```python
from build123d import *

# Parameters (mm, degrees)
SKETCH1_R           = 88.9
BOSS_EXTRUDE1_DEPTH = 76.2
CUT_EXTRUDE1_REACH  = 149.013


with BuildPart() as part:
    # Sketch1 → Boss-Extrude1 (new body)
    with BuildSketch(Plane.XY):
        with Locations(Location((0, 0, 0), (0, 0, 180))):
            Circle(SKETCH1_R)
    extrude(amount=BOSS_EXTRUDE1_DEPTH)

    # Sketch3 → Cut-Extrude1 (cut, up to next)
    with BuildSketch(Plane.XY.offset(76.2), mode=Mode.PRIVATE) as cut_extrude1_sk1:
        with BuildLine():
            Line((35.802288852, 13.030967461), (69.049928483, 32.226501152))
            ThreePointArc((69.049928483, 32.226501152), (74.391009371, 16.505081787), (76.2, 0))
            Line((76.2, 0), (38.1, 0))
            ThreePointArc((38.1, 0), (37.52117539, 6.615995569), (35.802288852, 13.030967461))
        make_face()
    cut_extrude1_tool1 = extrude(cut_extrude1_sk1.sketch, amount=-CUT_EXTRUDE1_REACH, mode=Mode.PRIVATE) & part.part
    # Sketch3 → Cut-Extrude1 (cut, up to next)
    with BuildSketch(Plane.XY.offset(76.2), mode=Mode.PRIVATE) as cut_extrude1_sk2:
        with BuildLine():
            Line((32.51038259, -19.866681249), (68.247619398, -33.892513133))
            ThreePointArc((68.247619398, -33.892513133), (59.286228254, -47.870482966), (47.509922902, -59.575558964))
            Line((47.509922902, -59.575558964), (23.754961451, -29.787779482))
            ThreePointArc((23.754961451, -29.787779482), (28.566663833, -25.210230412), (32.51038259, -19.866681249))
        make_face()
    cut_extrude1_tool2 = extrude(cut_extrude1_sk2.sketch, amount=-CUT_EXTRUDE1_REACH, mode=Mode.PRIVATE) & part.part
    # Sketch3 → Cut-Extrude1 (cut, up to next)
    with BuildSketch(Plane.XY.offset(76.2), mode=Mode.PRIVATE) as cut_extrude1_sk3:
        with BuildLine():
            Line((4.737495147, -37.804313771), (16.053460909, -74.489773747))
            ThreePointArc((16.053460909, -74.489773747), (-0.462291956, -76.198597665), (-16.956095167, -74.289506908))
            Line((-16.956095167, -74.289506908), (-8.478047584, -37.144753454))
            ThreePointArc((-8.478047584, -37.144753454), (-1.899128244, -38.052638698), (4.737495147, -37.804313771))
        make_face()
    cut_extrude1_tool3 = extrude(cut_extrude1_sk3.sketch, amount=-CUT_EXTRUDE1_REACH, mode=Mode.PRIVATE) & part.part
    # Sketch3 → Cut-Extrude1 (cut, up to next)
    with BuildSketch(Plane.XY.offset(76.2), mode=Mode.PRIVATE) as cut_extrude1_sk4:
        with BuildLine():
            Line((-26.602822769, -27.274526957), (-48.229281076, -58.994715415))
            ThreePointArc((-48.229281076, -58.994715415), (-59.862696895, -47.147614155), (-68.653827734, -33.061940921))
            Line((-68.653827734, -33.061940921), (-34.326913867, -16.53097046))
            ThreePointArc((-34.326913867, -16.53097046), (-30.934838018, -22.240633912), (-26.602822769, -27.274526957))
        make_face()
    cut_extrude1_tool4 = extrude(cut_extrude1_sk4.sketch, amount=-CUT_EXTRUDE1_REACH, mode=Mode.PRIVATE) & part.part
    # Sketch3 → Cut-Extrude1 (cut, up to next)
    with BuildSketch(Plane.XY.offset(76.2), mode=Mode.PRIVATE) as cut_extrude1_sk5:
        with BuildLine():
            Line((-37.910672541, 3.793534955), (-76.194390713, 0.924566897))
            ThreePointArc((-76.194390713, 0.924566897), (-74.185270095, 17.40648445), (-68.653827734, 33.061940921))
            Line((-68.653827734, 33.061940921), (-34.326913867, 16.53097046))
            ThreePointArc((-34.326913867, 16.53097046), (-36.675983809, 10.319021836), (-37.910672541, 3.793534955))
        make_face()
    cut_extrude1_tool5 = extrude(cut_extrude1_sk5.sketch, amount=-CUT_EXTRUDE1_REACH, mode=Mode.PRIVATE) & part.part
    # Sketch3 → Cut-Extrude1 (cut, up to next)
    with BuildSketch(Plane.XY.offset(76.2), mode=Mode.PRIVATE) as cut_extrude1_sk6:
        with BuildLine():
            Line((-20.671012653, 32.004987672), (-46.78357006, 60.147631478))
            ThreePointArc((-46.78357006, 60.147631478), (-32.64482181, 68.853145237), (-16.956095167, 74.289506908))
            Line((-16.956095167, 74.289506908), (-8.478047584, 37.144753454))
            ThreePointArc((-8.478047584, 37.144753454), (-14.799365738, 35.108243672), (-20.671012653, 32.004987672))
        make_face()
    cut_extrude1_tool6 = extrude(cut_extrude1_sk6.sketch, amount=-CUT_EXTRUDE1_REACH, mode=Mode.PRIVATE) & part.part
    # Sketch3 → Cut-Extrude1 (cut, up to next)
    with BuildSketch(Plane.XY.offset(76.2), mode=Mode.PRIVATE) as cut_extrude1_sk7:
        with BuildLine():
            Line((12.134341375, 36.116031889), (17.856233058, 74.078302768))
            ThreePointArc((17.856233058, 74.078302768), (33.477843131, 68.451983312), (47.509922902, 59.575558964))
            Line((47.509922902, 59.575558964), (23.754961451, 29.787779482))
            ThreePointArc((23.754961451, 29.787779482), (18.221476585, 33.460241945), (12.134341375, 36.116031889))
        make_face()
    cut_extrude1_tool7 = extrude(cut_extrude1_sk7.sketch, amount=-CUT_EXTRUDE1_REACH, mode=Mode.PRIVATE) & part.part
    add(cut_extrude1_tool1.solids().sort_by_distance((58.182027, 12.183187, 76.2))[0], mode=Mode.SUBTRACT)
    add(cut_extrude1_tool2.solids().sort_by_distance((45.8011, -37.892448, 76.2))[0], mode=Mode.SUBTRACT)
    add(cut_extrude1_tool3.solids().sort_by_distance((-1.06899, -59.434296, 76.2))[0], mode=Mode.SUBTRACT)
    add(cut_extrude1_tool4.solids().sort_by_distance((-47.134109, -36.220908, 76.2))[0], mode=Mode.SUBTRACT)
    add(cut_extrude1_tool5.solids().sort_by_distance((-57.706282, 14.267563, 76.2))[0], mode=Mode.SUBTRACT)
    add(cut_extrude1_tool6.solids().sort_by_distance((-24.824448, 54.012268, 76.2))[0], mode=Mode.SUBTRACT)
    add(cut_extrude1_tool7.solids().sort_by_distance((26.750702, 53.084633, 76.2))[0], mode=Mode.SUBTRACT)

    # Fillet2: read off the stored shape, not the designer's step
    # Fillet2 outline → Fillet2 (revolve, cut)
    with BuildSketch(Plane.XZ):
        with BuildLine():
            ThreePointArc((76.2, 76.2), (85.180256121, 72.480256121), (88.9, 63.5))
            Line((88.9, 63.5), (88.9, 76.2))
            Line((88.9, 76.2), (76.2, 76.2))
        make_face()
        with BuildLine():
            Line((88.9, 0), (88.9, 12.7))
            ThreePointArc((88.9, 12.7), (85.180256121, 3.719743879), (76.2, 0))
            Line((76.2, 0), (88.9, 0))
        make_face()
    revolve(axis=Axis((0, 0, 0), (0, 0, 1)), mode=Mode.SUBTRACT)


solid = part.part
```
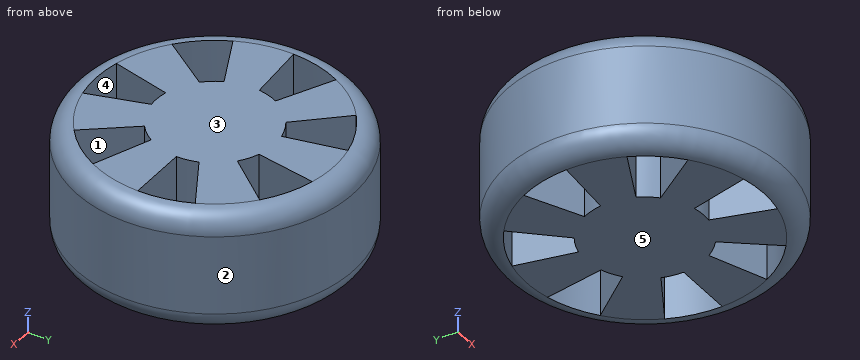
Geometry check sheet. Reference: the model listing, model coordinates, mm. Face numbers are marked on the shaded views. A direction names the side the tool comes from. Round coordinates to 2 decimals unless told otherwise and drop trailing zeros. Loops run counter-clockwise (first coordinate to the right, second up) from the corner with the lowest first, then second, coordinate; pieces in that order, holes last. Notation, with made-up numbers: (51.5, 66) - (82.5, 66) arc R26 ccw to (82.5, 86) - close; hole circle Ø1 at (7.25, -5.75). An arc over 180 degrees is marked (long way). Write each question's results on one line, items separated by ' | '. Start each with the question number.
Q1. Access from +Z, -Z, +X, -X, +Y, -Y to the whole of each face (thin tool, end or side, straight path). Record for the marked faces 4 and 5.
Q2. Cross-section at A-A on z = 43. State how many separate pieces and enclosed holes the cut face has, and give its area (3 significant figures).
Q3. Gauge pin test, flat ends, axial feed: P1, Ø2, axis at x = 51, z = 49.5, coming from the +Y side; P2, Ø4, axis at x = 4.5, z = 24, coming from the +Y side; P3, Ø1.5, axis at x = -57, z = 21.5, coming from the +Y side. Record the tip position at first contact, or that the pin passes through.
Q4. Thickness scan on line 1 (X direction, y = 39, z = 16); line 2 (X direction, y = 38, z = 49.5); line 3 (Y direction, x = -32.5, z = 63). Record the ranges inside material, lowest first. Write a range as [from, to].
Q5. Cross-section at B-B on x = 0. Enter the section's corners in (y, z).
Q6. Release check for a two-part mould opening along Y. For the marked faces 1, 2 and 3 record: +Y half, -Y half, draft (parallel to the pull), parting line (faces both ways), or undercut.
Answers below:
1) face 4: +Z, -Z | face 5: -Z, +X, -X, +Y, -Y
2) separate pieces: 1 | enclosed holes: 7 | area: 18,600 mm²
3) P1: stops at y = 73.51 | P2: stops at y = 88.86 | P3: stops at y = 68.84
4) line 1: x = [-79.89, -27.16], [-8.9, 12.57], [31.1, 79.89] | line 2: x = [-80.37, -26.23], [-8.67, 12.42], [30.3, 80.37] | line 3: y = [-82.75, -35.92], [-19.88, 44.75], [68.92, 82.75]
5) outline: (-88.9, 12.7) arc R12.7 ccw to (-76.2, 0) - (-76.2, 76.2) arc R12.7 ccw to (-88.9, 63.5) - close; (-38.1, 0) - (76.2, 0) arc R12.7 ccw to (88.9, 12.7) - (88.9, 63.5) arc R12.7 ccw to (76.2, 76.2) - (-38.1, 76.2) - close
6) face 1: undercut | face 2: parting line | face 3: draft
